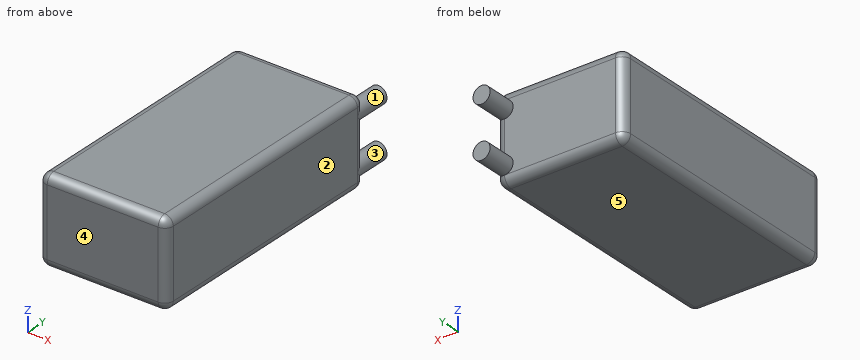
from build123d import *

# Parameters (mm, degrees)
SKETCH1_W           = 30
SKETCH1_H           = 20
BOSS_EXTRUDE1_DEPTH = 60
SKETCH2_R           = 2
BOSS_EXTRUDE2_DEPTH = 7
FILLET1_R           = 2


with BuildPart() as part:
    # Sketch1 → Boss-Extrude1 (new body)
    with BuildSketch(Plane(origin=(0, 0, 0), x_dir=(1, 0, 0), z_dir=(0, 1, 0))):
        Rectangle(SKETCH1_W, SKETCH1_H)
    extrude(amount=BOSS_EXTRUDE1_DEPTH)

    # Sketch2 → Boss-Extrude2 (add)
    with BuildSketch(Plane(origin=(0, 60, 0), x_dir=(1, 0, 0), z_dir=(0, 1, 0))):
        with Locations((13, 6)):
            Circle(SKETCH2_R)
        with Locations((13, -6)):
            Circle(SKETCH2_R)
    extrude(amount=BOSS_EXTRUDE2_DEPTH)

    # Fillet1
    # the kernel refuses this fillet: 2 mm, written as the material it takes off along each edge
    with BuildSketch(Plane(origin=(13, 58, 8), x_dir=(0, 1, 0), z_dir=(1, 0, 0))) as fillet1_piece_1_section:
        Polygon((0, 0), (FILLET1_R * 1.02, 0), (FILLET1_R * 1.02, FILLET1_R * 1.02), (0, FILLET1_R * 1.02), align=None)
    fillet1_piece_1 = extrude(amount=FILLET1_R * 1.02, mode=Mode.PRIVATE)
    fillet1_piece_1 = fillet1_piece_1 - Plane(origin=(13, 58, 8), x_dir=(0, -0.7071067811865475, -0.7071067811865475), z_dir=(1, 0, 0)) * Sphere(FILLET1_R, mode=Mode.PRIVATE)
    add(fillet1_piece_1, mode=Mode.SUBTRACT)
    with BuildSketch(Plane(origin=(13, 58, -8), x_dir=(1, 0, 0), z_dir=(0, 0, -1))) as fillet1_piece_2_section:
        Polygon((0, 0), (FILLET1_R * 1.02, 0), (FILLET1_R * 1.02, -FILLET1_R * 1.02), (0, -FILLET1_R * 1.02), align=None)
    fillet1_piece_2 = extrude(amount=FILLET1_R * 1.02, mode=Mode.PRIVATE)
    fillet1_piece_2 = fillet1_piece_2 - Plane(origin=(13, 58, -8), x_dir=(-0.7071067811865475, -0.7071067811865475, 0), z_dir=(0, 0, -1)) * Sphere(FILLET1_R, mode=Mode.PRIVATE)
    add(fillet1_piece_2, mode=Mode.SUBTRACT)
    with BuildSketch(Plane(origin=(-13, 58, -8), x_dir=(-1, 0, 0), z_dir=(0, 0, -1))) as fillet1_piece_3_section:
        Polygon((0, 0), (FILLET1_R * 1.02, 0), (FILLET1_R * 1.02, FILLET1_R * 1.02), (0, FILLET1_R * 1.02), align=None)
    fillet1_piece_3 = extrude(amount=FILLET1_R * 1.02, mode=Mode.PRIVATE)
    fillet1_piece_3 = fillet1_piece_3 - Plane(origin=(-13, 58, -8), x_dir=(0.7071067811865475, -0.7071067811865475, 0), z_dir=(0, 0, -1)) * Sphere(FILLET1_R, mode=Mode.PRIVATE)
    add(fillet1_piece_3, mode=Mode.SUBTRACT)
    with BuildSketch(Plane(origin=(-13, 58, 8), x_dir=(0, 1, 0), z_dir=(-1, 0, 0))) as fillet1_piece_4_section:
        Polygon((0, 0), (FILLET1_R * 1.02, 0), (FILLET1_R * 1.02, -FILLET1_R * 1.02), (0, -FILLET1_R * 1.02), align=None)
    fillet1_piece_4 = extrude(amount=FILLET1_R * 1.02, mode=Mode.PRIVATE)
    fillet1_piece_4 = fillet1_piece_4 - Plane(origin=(-13, 58, 8), x_dir=(0, -0.7071067811865475, -0.7071067811865475), z_dir=(-1, 0, 0)) * Sphere(FILLET1_R, mode=Mode.PRIVATE)
    add(fillet1_piece_4, mode=Mode.SUBTRACT)
    with BuildSketch(Plane(origin=(13, 2, -8), x_dir=(1, 0, 0), z_dir=(0, 0, -1))) as fillet1_piece_5_section:
        Polygon((0, 0), (FILLET1_R * 1.02, 0), (FILLET1_R * 1.02, FILLET1_R * 1.02), (0, FILLET1_R * 1.02), align=None)
    fillet1_piece_5 = extrude(amount=FILLET1_R * 1.02, mode=Mode.PRIVATE)
    fillet1_piece_5 = fillet1_piece_5 - Plane(origin=(13, 2, -8), x_dir=(-0.7071067811865475, 0.7071067811865475, 0), z_dir=(0, 0, -1)) * Sphere(FILLET1_R, mode=Mode.PRIVATE)
    add(fillet1_piece_5, mode=Mode.SUBTRACT)
    with BuildSketch(Plane(origin=(-13, 2, -8), x_dir=(-1, 0, 0), z_dir=(0, 0, -1))) as fillet1_piece_6_section:
        Polygon((0, 0), (FILLET1_R * 1.02, 0), (FILLET1_R * 1.02, -FILLET1_R * 1.02), (0, -FILLET1_R * 1.02), align=None)
    fillet1_piece_6 = extrude(amount=FILLET1_R * 1.02, mode=Mode.PRIVATE)
    fillet1_piece_6 = fillet1_piece_6 - Plane(origin=(-13, 2, -8), x_dir=(0.7071067811865475, 0.7071067811865475, 0), z_dir=(0, 0, -1)) * Sphere(FILLET1_R, mode=Mode.PRIVATE)
    add(fillet1_piece_6, mode=Mode.SUBTRACT)
    with BuildSketch(Plane(origin=(13, 2, 8), x_dir=(0, -1, 0), z_dir=(1, 0, 0))) as fillet1_piece_7_section:
        Polygon((0, 0), (FILLET1_R * 1.02, 0), (FILLET1_R * 1.02, -FILLET1_R * 1.02), (0, -FILLET1_R * 1.02), align=None)
    fillet1_piece_7 = extrude(amount=FILLET1_R * 1.02, mode=Mode.PRIVATE)
    fillet1_piece_7 = fillet1_piece_7 - Plane(origin=(13, 2, 8), x_dir=(0, 0.7071067811865475, -0.7071067811865475), z_dir=(1, 0, 0)) * Sphere(FILLET1_R, mode=Mode.PRIVATE)
    add(fillet1_piece_7, mode=Mode.SUBTRACT)
    with BuildSketch(Plane(origin=(-13, 2, 8), x_dir=(0, -1, 0), z_dir=(-1, 0, 0))) as fillet1_piece_8_section:
        Polygon((0, 0), (FILLET1_R * 1.02, 0), (FILLET1_R * 1.02, FILLET1_R * 1.02), (0, FILLET1_R * 1.02), align=None)
    fillet1_piece_8 = extrude(amount=FILLET1_R * 1.02, mode=Mode.PRIVATE)
    fillet1_piece_8 = fillet1_piece_8 - Plane(origin=(-13, 2, 8), x_dir=(0, 0.7071067811865475, -0.7071067811865475), z_dir=(-1, 0, 0)) * Sphere(FILLET1_R, mode=Mode.PRIVATE)
    add(fillet1_piece_8, mode=Mode.SUBTRACT)
    with BuildSketch(Plane(origin=(15, 60, 8), x_dir=(0, -1, 0), z_dir=(0, 0, -1))) as fillet1_piece_9_section:
        with BuildLine():
            CenterArc((FILLET1_R, FILLET1_R), FILLET1_R, 180, 90)
            Line((0, FILLET1_R), (0, 0))
            Line((0, 0), (FILLET1_R, 0))
        make_face()
    fillet1_piece_9 = extrude(amount=2, mode=Mode.PRIVATE)
    fillet1_piece_9 = fillet1_piece_9 - Plane(origin=(13, 59.42884434, 6), x_dir=(1, 0, 0), z_dir=(0, -1, 0)) * Cylinder(2, 12, mode=Mode.PRIVATE)
    add(fillet1_piece_9, mode=Mode.SUBTRACT)
    with BuildSketch(Plane(origin=(15, 60, -6), x_dir=(0, -1, 0), z_dir=(0, 0, -1))) as fillet1_piece_10_section:
        with BuildLine():
            CenterArc((FILLET1_R, FILLET1_R), FILLET1_R, 180, 90)
            Line((0, FILLET1_R), (0, 0))
            Line((0, 0), (FILLET1_R, 0))
        make_face()
    fillet1_piece_10 = extrude(amount=2, mode=Mode.PRIVATE)
    fillet1_piece_10 = fillet1_piece_10 - Plane(origin=(13, 59.42884434, -6), x_dir=(1, 0, 0), z_dir=(0, -1, 0)) * Cylinder(2, 13, mode=Mode.PRIVATE)
    add(fillet1_piece_10, mode=Mode.SUBTRACT)
    with BuildSketch(Plane(origin=(13, 60, -10), x_dir=(0, -1, 0), z_dir=(-1, 0, 0)), Plane(origin=(-13, 0, 10), x_dir=(0, 0, -1), z_dir=(1, 0, 0))) as fillet1_piece_11:
        with BuildLine():
            CenterArc((FILLET1_R, FILLET1_R), FILLET1_R, 180, 90)
            Line((0, FILLET1_R), (0, 0))
            Line((0, 0), (FILLET1_R, 0))
        make_face()
    extrude(amount=26, mode=Mode.SUBTRACT)
    with BuildSketch(Plane(origin=(15, 60, 6), x_dir=(0, -1, 0), z_dir=(0, 0, -1))) as fillet1_piece_12_section:
        with BuildLine():
            CenterArc((FILLET1_R, FILLET1_R), FILLET1_R, 180, 90)
            Line((0, FILLET1_R), (0, 0))
            Line((0, 0), (FILLET1_R, 0))
        make_face()
    fillet1_piece_12 = extrude(amount=12, mode=Mode.PRIVATE)
    fillet1_piece_12 = fillet1_piece_12 - Plane(origin=(13, 59.530547013, 6), x_dir=(1, 0, 0), z_dir=(0, -1, 0)) * Cylinder(2, 32, mode=Mode.PRIVATE)
    fillet1_piece_12 = fillet1_piece_12 - Plane(origin=(13, 59.530547013, -6), x_dir=(1, 0, 0), z_dir=(0, -1, 0)) * Cylinder(2, 32, mode=Mode.PRIVATE)
    add(fillet1_piece_12, mode=Mode.SUBTRACT)
    with BuildSketch(Plane(origin=(-15, 60, -8), x_dir=(0, -1, 0), z_dir=(0, 0, 1))) as fillet1_piece_13:
        with BuildLine():
            CenterArc((FILLET1_R, FILLET1_R), FILLET1_R, 180, 90)
            Line((0, FILLET1_R), (0, 0))
            Line((0, 0), (FILLET1_R, 0))
        make_face()
    extrude(amount=16, mode=Mode.SUBTRACT)
    with BuildSketch(Plane(origin=(13, 0, -10), x_dir=(0, 1, 0), z_dir=(-1, 0, 0)), Plane(origin=(-13, 60, 10), x_dir=(0, 0, -1), z_dir=(1, 0, 0))) as fillet1_piece_14:
        with BuildLine():
            CenterArc((FILLET1_R, -FILLET1_R), FILLET1_R, 90, 90)
            Line((0, -FILLET1_R), (0, 0))
            Line((0, 0), (FILLET1_R, 0))
        make_face()
    extrude(amount=26, mode=Mode.SUBTRACT)
    with BuildSketch(Plane(origin=(15, 0, 8), x_dir=(0, 1, 0), z_dir=(0, 0, -1)), Plane(origin=(-15, 0, -8), x_dir=(0, 1, 0), z_dir=(0, 0, 1))) as fillet1_piece_15:
        with BuildLine():
            CenterArc((FILLET1_R, -FILLET1_R), FILLET1_R, 90, 90)
            Line((0, -FILLET1_R), (0, 0))
            Line((0, 0), (FILLET1_R, 0))
        make_face()
    extrude(amount=16, mode=Mode.SUBTRACT)
    with BuildSketch(Plane(origin=(-15, 2, -10), x_dir=(1, 0, 0), z_dir=(0, 1, 0)), Plane(origin=(-15, 2, 10), x_dir=(0, 0, -1), z_dir=(0, 1, 0))) as fillet1_piece_16:
        with BuildLine():
            CenterArc((FILLET1_R, -FILLET1_R), FILLET1_R, 90, 90)
            Line((0, -FILLET1_R), (0, 0))
            Line((0, 0), (FILLET1_R, 0))
        make_face()
    extrude(amount=56, mode=Mode.SUBTRACT)
    with BuildSketch(Plane(origin=(15, 2, -10), x_dir=(-1, 0, 0), z_dir=(0, 1, 0)), Plane(origin=(15, 2, 10), x_dir=(0, 0, -1), z_dir=(0, 1, 0))) as fillet1_piece_17:
        with BuildLine():
            CenterArc((FILLET1_R, FILLET1_R), FILLET1_R, 180, 90)
            Line((0, FILLET1_R), (0, 0))
            Line((0, 0), (FILLET1_R, 0))
        make_face()
    extrude(amount=56, mode=Mode.SUBTRACT)


solid = part.part
Build history of the part. All positions in model axes, mm. Face numbers are marked on the shaded views. A direction names the side the tool comes from. Round coordinates to 2 decimals unless told otherwise and drop trailing zeros. Write each loop counter-clockwise with the first axis right and the second up, starting at its lowest first coordinate (ties: lowest second). Pieces come first, ordered by that corner, then holes. Notation, with made-up numbers: M 31,8 L 58,8 A30 ccw 58,38 Z; hole C 16,-25.5 d1. An arc over 180 degrees is marked long. Use CSV: the item, a comma, the result in double quotes.
1. Saw through at C-C (z = 7). Give the cut face in (x, y).
Reply:
outline,"M -15,2 A2 ccw -13,0 L 13,0 A2 ccw 15,2 L 15,58 A2 ccw 14.73,59 L 14.73,67 L 11.27,67 L 11.27,60 L -13,60 A2 ccw -15,58 Z"
2. Flat gauge pin, fed straight in: pin 1 (8 mm diameter, centred on x = 2.5, z = 3, fed in from +Y). Where does the tip first touch, or does it go through?
Reply:
pin 1,"stops at y = 60"
3. Two-plate mould, pull along Z, no slides. Class the marked faces 3, 4 and 5: +Z half, -Z half, draft (parallel to the pull), parting line (faces both ways), or undercut.
Reply:
face 3,"undercut"
face 4,"draft"
face 5,"-Z half"
4. Tool access for the marked faces 1 and 2: list every direction of +Z, -Z, +X, -X, +Y, -Y with a clear straight run to the whole face (end or side of a thin tool).
Reply:
face 1,"+Y"
face 2,"+Z, -Z, +X, +Y, -Y"
5. Saw through at B-B (z = -3). Give the cut face in (x, y).
Reply:
outline,"M -15,2 A2 ccw -13,0 L 13,0 A2 ccw 15,2 L 15,58 A2 ccw 13,60 L -13,60 A2 ccw -15,58 Z"
6. Wall check: probe 1 along Y at (x, z) = (10, 7.75); probe 2 along Y at (x, z) = (1.5, 8.5); probe 3 along X at (y, z) = (59, 4.75). Give the ranges that are in metal, low to high. Write a range as from..to.
Reply:
probe 1,"y = 0..60"
probe 2,"y = 0.06..59.94"
probe 3,"x = -14.73..14.73"
7. Saw through at A-A (x = 10). Give the cut face in (y, z).
Reply:
outline,"M 0,-8 A2 ccw 2,-10 L 58,-10 A2 ccw 60,-8 L 60,8 A2 ccw 58,10 L 2,10 A2 ccw 0,8 Z"
